Build history of the part. All positions in model axes, mm. Face numbers are marked on the shaded views. A direction names the side the tool comes from. Round coordinates to 2 decimals unless told otherwise and drop trailing zeros. Write each loop counter-clockwise with the first axis right and the second up, starting at its lowest first coordinate (ties: lowest second). Pieces come first, ordered by that corner, then holes.
Item 1: Mould opens along X. For the marked faces 1, 2 and 3 say: +X half, -X half, draft (parallel to the pull), parting line (faces both ways), or undercut.
Item 2: Band-saw the part on C-C, the plane z = 27. Write the cut outline in (x, y).
Item 3: Band-saw the part on B-B, the plane y = 8. Write the cut outline in (x, z), then the cut area to 3 significant figures.
Item 4: 3-axis set-ups, long thin cutter, end or side, ignore diameter. For the marked faces 4, 5, 6 and 7: which of +Z, -Z, +X, -X, +Y, -Y reach the whole face in a straight line?
Item 5: Drop flat-ended pins along their axis: pin 1 Ø1 at (y, z) = (27.5, 38.5) entering from +X; pin 2 Ø8 at (x, y) = (-58.5, 2.5) entering from +Z; pin 3 Ø8 at (x, y) = (-35, 41) entering from -Z. Give the stop position or say it passes through.
Item 6: Wall check: probe 1 along X at (y, z) = (5, 5); probe 2 along Z at (x, y) = (21.5, 11.5); probe 3 along Y at (x, z) = (67, 3). Give the ranges that are in metal, low to high.
Item 7: Band-saw the part on A-A, the plane x = -23.5. Write the cut outline in (y, z).
Item 8: Band-saw the part on D-D, the plane y = 30. Write the cut outline in (x, z).
```python
from build123d import *

# Parameters (mm, degrees)
SKETCH_W        = 150
SKETCH_H        = 100
PAD_DEPTH       = 50
SKETCH001_R     = 3.5
PAD001_DEPTH    = 5
SKETCH002_W     = 33
SKETCH002_H     = 12
POCKET_DEPTH    = 20
FILLET_R        = 29
SKETCH004_W     = 126
SKETCH004_H     = 76
POCKET001_DEPTH = 25
SKETCH005_R     = 4
POCKET002_DEPTH = 5
SKETCH006_W     = 20.5
SKETCH006_H     = 20
POCKET003_DEPTH = 100
SKETCH008_W     = 16
SKETCH008_H     = 21
POCKET004_DEPTH = 200


with BuildPart() as part:
    # Sketch → Pad (new body)
    with BuildSketch(Plane.XY):
        Rectangle(SKETCH_W, SKETCH_H)
    extrude(amount=PAD_DEPTH)

    # Sketch001 (on Face5 of Pad) → Pad001 (join)
    with BuildSketch(Plane(origin=(0, 0, 0), x_dir=(1, 0, 0), z_dir=(0, 0, -1))):
        with Locations((67.5, 30)):
            Circle(SKETCH001_R)
        with Locations((67.5, -30)):
            Circle(SKETCH001_R)
        with Locations((-67.5, -30)):
            Circle(SKETCH001_R)
        with Locations((-67.5, 30)):
            Circle(SKETCH001_R)
    extrude(amount=PAD001_DEPTH)

    # Sketch002 (on Face4 of Pad001) → Pocket (cut)
    with BuildSketch(Plane(origin=(0, 0, 0), x_dir=(1, 0, 0), z_dir=(0, 0, -1))):
        with Locations((-53.5, 44)):
            Rectangle(SKETCH002_W, SKETCH002_H)
        with Locations((53.5, 44)):
            Rectangle(SKETCH002_W, SKETCH002_H)
        with Locations((0, 44)):
            Rectangle(SKETCH002_W, SKETCH002_H)
        with Locations((-53.5, -44)):
            Rectangle(SKETCH002_W, SKETCH002_H)
        with Locations((0, -44)):
            Rectangle(SKETCH002_W, SKETCH002_H)
        with Locations((53.5, -44)):
            Rectangle(SKETCH002_W, SKETCH002_H)
    extrude(amount=-POCKET_DEPTH, mode=Mode.SUBTRACT)

    # Fillet
    fillet_edges = [part.edges().sort_by_distance(p)[0] for p in [
        (0, 50, 50),
        (75, 0, 50),
        (0, -50, 50),
        (-75, 0, 50),
    ]]
    fillet(fillet_edges, radius=FILLET_R)

    # Sketch004 (on Face4 of Fillet) → Pocket001 (cut)
    with BuildSketch(Plane(origin=(0, 0, 0), x_dir=(1, 0, 0), z_dir=(0, 0, -1))):
        Rectangle(SKETCH004_W, SKETCH004_H)
    extrude(amount=-POCKET001_DEPTH, mode=Mode.SUBTRACT)

    # Sketch005 (on Face12 of Pocket001) → Pocket002 (cut)
    with BuildSketch(Plane(origin=(0, 0, 0), x_dir=(1, 0, 0), z_dir=(0, 0, -1))):
        with Locations((-26, 42.5)):
            Circle(SKETCH005_R)
        with Locations((27.5, 42.5)):
            Circle(SKETCH005_R)
        with Locations((-26, -42.5)):
            Circle(SKETCH005_R)
        with Locations((27.5, -42.5)):
            Circle(SKETCH005_R)
    extrude(amount=-POCKET002_DEPTH, mode=Mode.SUBTRACT)

    # Sketch006 (on Face19 of Pocket002) → Pocket003 (cut)
    with BuildSketch(Plane.XZ.offset(50)):
        with Locations((-26.75, 10)):
            Rectangle(SKETCH006_W, SKETCH006_H)
        with Locations((26.75, 10)):
            Rectangle(SKETCH006_W, SKETCH006_H)
    extrude(amount=-POCKET003_DEPTH, mode=Mode.SUBTRACT)

    # Sketch008 (on Face3 of Pocket003) → Pocket004 (cut)
    with BuildSketch(Plane(origin=(-75, 0, 0), x_dir=(0, -1, 0), z_dir=(-1, 0, 0))):
        with Locations((-42, 10.5)):
            Rectangle(SKETCH008_W, SKETCH008_H)
        with Locations((42, 10.5)):
            Rectangle(SKETCH008_W, SKETCH008_H)
    extrude(amount=-POCKET004_DEPTH, mode=Mode.SUBTRACT)


solid = part.part
```
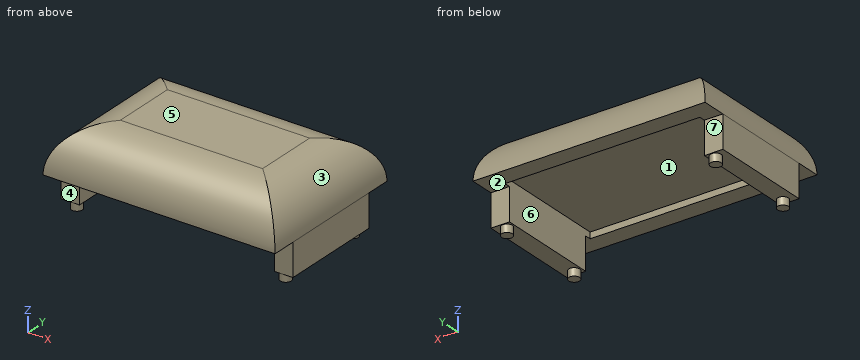
Results:
1. face 1: undercut
1. face 2: draft
1. face 3: +X half
2. outline: (-74.37, -49.37) - (74.37, -49.37) - (74.37, 49.37) - (-74.37, 49.37) - close
3. outline: (-75, 0) - (-63, 0) - (-63, 25) - (63, 25) - (63, 0) - (75, 0) - (75, 21) arc R29 ccw to (46, 50) - (-46, 50) arc R29 ccw to (-75, 21) - close
3. area: 3,990 mm2
4. face 4: -Z, +X, -X, -Y
4. face 5: +Z, +X, -X, +Y, -Y
4. face 6: -Z
4. face 7: -Z, +X, -X, +Y
5. pin 1: stops at x = 69.49
5. pin 2: stops at z = 48.73
5. pin 3: stops at z = 21
6. probe 1: x = -75 to -63, 63 to 75
6. probe 2: z = 25 to 50
6. probe 3: y = -34 to 34
7. outline: (-50, 21) - (-38, 21) - (-38, 25) - (38, 25) - (38, 21) - (50, 21) arc R29 ccw to (21, 50) - (-21, 50) arc R29 ccw to start
8. outline: (-75, 0) - (-71, 0) - (-71, -5) - (-64, -5) - (-64, 0) - (-63, 0) - (-63, 25) - (63, 25) - (63, 0) - (64, 0) - (64, -5) - (71, -5) - (71, 0) - (75, 0) - (75, 21) arc R29 ccw to (55, 48.57) - (-55, 48.57) arc R29 ccw to (-75, 21) - close
